from build123d import *

# Parameters (mm, degrees)
SKETCH_W        = 37
SKETCH_H        = 37
PAD_DEPTH       = 4
SKETCH001_R     = 1.75
POCKET_DEPTH    = 4.001
SKETCH002_W     = 8
SKETCH002_H     = 8
POCKET001_DEPTH = 2


with BuildPart() as part:
    # Sketch → Pad (new body)
    with BuildSketch(Plane.XY):
        Rectangle(SKETCH_W, SKETCH_H)
    extrude(amount=PAD_DEPTH)

    # Sketch001 (on Face6 of Pad) → Pocket (cut, through all)
    with BuildSketch(Plane.XY.offset(4)):
        with Locations((-15, 15)):
            Circle(SKETCH001_R)
        with Locations((15, 15)):
            Circle(SKETCH001_R)
        with Locations((-15, -15)):
            Circle(SKETCH001_R)
        with Locations((15, -15)):
            Circle(SKETCH001_R)
    extrude(amount=-POCKET_DEPTH, mode=Mode.SUBTRACT)

    # Sketch002 (on Face5 of Pocket) → Pocket001 (cut)
    with BuildSketch(Plane.XY.offset(4)):
        with Locations((-14.5, 14.5)):
            Rectangle(SKETCH002_W, SKETCH002_H)
        with Locations((14.5, 14.5)):
            Rectangle(SKETCH002_W, SKETCH002_H)
        with Locations((14.5, -14.5)):
            Rectangle(SKETCH002_W, SKETCH002_H)
        with Locations((-14.5, -14.5)):
            Rectangle(SKETCH002_W, SKETCH002_H)
    extrude(amount=-POCKET001_DEPTH, mode=Mode.SUBTRACT)


solid = part.part
Model file for the job. Use its own axes, mm. A direction names the side the tool comes from. Give positions to 0.01 mm unless a question says otherwise; leave off trailing zeros. Loops run counter-clockwise (first coordinate to the right, second up) from the corner with the lowest first, then second, coordinate; pieces in that order, holes last. Notation, with made-up numbers: (-19, 33) -> (-4, 33) arc R33 cw to (-4, 71) -> close; hole circle Ø10 at (-27.5, 40.5). An arc over 180 degrees is marked (long way). Use a Markdown table: item, result. Add a question column.
(1) Mould opens along X. For faces 1 (the flat face through (14, -10.5, 3)), 2 (the flat face through (10.5, 14, 3)), 3 (the cylindrical face through (14.772, 16.735, 1.014)) say: +X half, -X half, draft (parallel to the pull), parting line (faces both ways), or undercut.
(2) Slice it at D-D on z = 2.65. List the corners of the cut face in (x, y).
(3) Slice it at A-A on y = -15. List the corners of the cut face in (x, z).
(4) Slice it at C-C on z = 0.8. List the corners of the cut face in (x, y), and give its area (3 significant figures).
(5) Tool access for faces 4 (the flat face through (13.6, -13.6, 2)), 5 (the flat face through (-15, 13, 2)), 6 (the flat face through (-10.5, -15, 3)), 7 (the flat face through (13.6, 13.7, 2)): list every direction of +Z, -Z, +X, -X, +Y, -Y with a clear straight run to the whole face (end or side of a thin tool).
(6) Wall check: line 1 along Y through (x, z) = (15, 0.85); line 2 along Y through (x, z) = (-13.5, 0.6); line 3 along Y through (x, z) = (11, 3.6). Give the ranges that are in metal, low to high.
(7) Drop flat-ended pins along their axis: pin 1 Ø4 at (x, y) = (16.5, -13) entering from +Z; pin 2 Ø1 at (y, z) = (-13, 3) entering from -X; pin 3 Ø0.6 at (x, z) = (-13, 3.5) entering from -Y. Give the stop position or say it passes through.
Filled sheet:
| question | item | result |
|---|---|---|
| 1 | face 1 | draft |
| 1 | face 2 | +X half |
| 1 | face 3 | undercut |
| 2 | outline | (-18.5, -10.5) -> (-10.5, -10.5) -> (-10.5, -18.5) -> (10.5, -18.5) -> (10.5, -10.5) -> (18.5, -10.5) -> (18.5, 10.5) -> (10.5, 10.5) -> (10.5, 18.5) -> (-10.5, 18.5) -> (-10.5, 10.5) -> (-18.5, 10.5) -> close |
| 3 | outline | (-18.5, 0) -> (-16.75, 0) -> (-16.75, 2) -> (-18.5, 2) -> close; (-13.25, 0) -> (13.25, 0) -> (13.25, 2) -> (10.5, 2) -> (10.5, 4) -> (-10.5, 4) -> (-10.5, 2) -> (-13.25, 2) -> close; (16.75, 0) -> (18.5, 0) -> (18.5, 2) -> (16.75, 2) -> close |
| 4 | outline | (-18.5, -18.5) -> (18.5, -18.5) -> (18.5, 18.5) -> (-18.5, 18.5) -> close; hole circle Ø3.5 at (-15, -15); hole circle Ø3.5 at (-15, 15); hole circle Ø3.5 at (15, -15); hole circle Ø3.5 at (15, 15) |
| 4 | area | 1,330 mm2 |
| 5 | face 4 | +Z, +X, -Y |
| 5 | face 5 | +Z, -X, +Y |
| 5 | face 6 | +Z, -X, -Y |
| 5 | face 7 | +Z, +X, +Y |
| 6 | line 1 | -18.5 to -16.75, -13.25 to 13.25, 16.75 to 18.5 |
| 6 | line 2 | -18.5 to -15.9, -14.1 to 14.1, 15.9 to 18.5 |
| 6 | line 3 | -10.5 to 10.5 |
| 7 | pin 1 | z = 2 |
| 7 | pin 2 | x = -10.5 |
| 7 | pin 3 | y = -10.5 |
